The drawing under review shows one solid part. Ordinate dimensions are in mm from its lowest x, y, z. A direction names the side the tool comes from. Give positions to 0.01 mm unless a question says otherwise; leave off trailing zeros. Order: outer loops, then holes, each group sorted by start corner. A loop starts at its lowest first (then second) coordinate and runs counter-clockwise, first axis right, second up. Notation, with made-up numbers: (52.25, 0.5) - (77.25, 0.5) arc R3 ccw to (77.25, 5.5) - close; hole circle Ø9 at (73, 0.5). An arc over 180 degrees is marked (long way). Use CSV: the item, a comma, the result in double quotes.
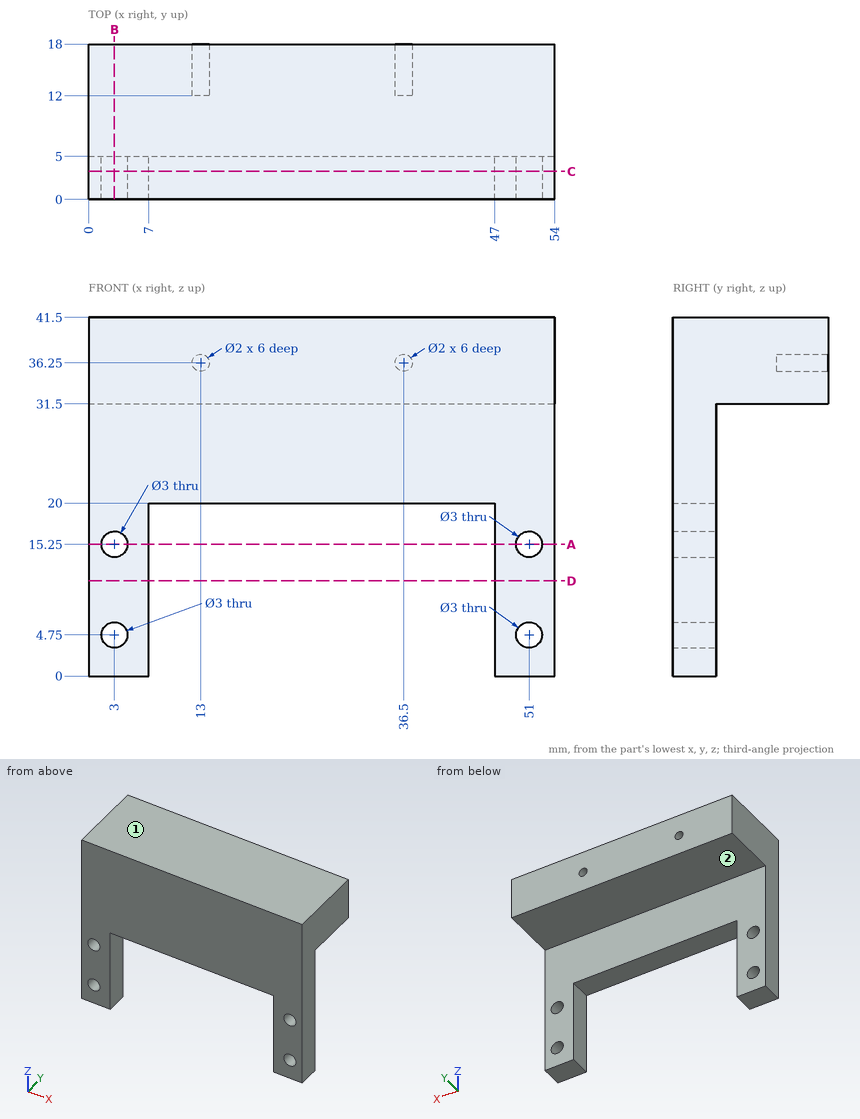
Item 1: Take a section at A-A, the plane z = 15.25. Give the boundary of the cut face in (x, y).
Results list:
outline,"(0, 0) - (1.5, 0) - (1.5, 5) - (0, 5) - close; (4.5, 0) - (7, 0) - (7, 5) - (4.5, 5) - close; (47, 0) - (49.5, 0) - (49.5, 5) - (47, 5) - close; (52.5, 0) - (54, 0) - (54, 5) - (52.5, 5) - close"
Item 2: Take a section at D-D, the plane z = 11. Give the boundary of the cut face in (x, y).
Results list:
outline,"(0, 0) - (7, 0) - (7, 5) - (0, 5) - close; (47, 0) - (54, 0) - (54, 5) - (47, 5) - close"
Item 3: Take a section at B-B, the plane x = 3. Give the boundary of the cut face in (y, z), and give its area (4 significant figures).
Results list:
outline,"(0, 0) - (5, 0) - (5, 3.25) - (0, 3.25) - close; (0, 6.25) - (5, 6.25) - (5, 13.75) - (0, 13.75) - close; (0, 16.75) - (5, 16.75) - (5, 31.5) - (18, 31.5) - (18, 41.5) - (0, 41.5) - close"
area,"307.5 mm2"
Item 4: Take a section at C-C, the plane y = 3.25. Give the boundary of the cut face in (x, z).
Results list:
outline,"(0, 0) - (7, 0) - (7, 20) - (47, 20) - (47, 0) - (54, 0) - (54, 41.5) - (0, 41.5) - close; hole circle Ø3 at (3, 4.75); hole circle Ø3 at (3, 15.25); hole circle Ø3 at (51, 4.75); hole circle Ø3 at (51, 15.25)"
Item 5: Tool access review of the marked faces 1 and 2: name each direction out of +Z, -Z, +X, -X, +Y, -Y from which nothing blocks a thin tool from reaching the whole face with its end or side.
Results list:
face 1,"+Z, +X, -X, +Y, -Y"
face 2,"-Z, +X, -X, +Y"
Item 6: Wall thickness on L1, parallel to X at y = 2.8, z = 15.25; L2, parallel to Z at x = 51, y = 2.8; L3, parallel to X at y = 16.45, z = 36.25: over which ranges is each line inside the solid? List them lowest first.
Results list:
L1,"x = 0 to 1.5, 4.5 to 7, 47 to 49.5, 52.5 to 54"
L2,"z = 0 to 3.25, 6.25 to 13.75, 16.75 to 41.5"
L3,"x = 0 to 12, 14 to 35.5, 37.5 to 54"
Item 7: Clearance check with flat-ended pins moving along their axes: pin 1 (4 mm diameter, centred on x = 3, z = 15.25, fed in from +Y); pin 2 (10 mm diameter, centred on x = 39.5, y = 3.5, fed in from -Z); pin 3 (1 mm diameter, centred on x = 13, z = 36, fed in from +Y). State where each tip first meets the part, or that it passes through.
Results list:
pin 1,"stops at y = 5"
pin 2,"stops at z = 20"
pin 3,"stops at y = 12"
